Can you work these out from the drawing? Everything is in mm from the part's minimum corner. A direction names the side the tool comes from. Give positions to 0.01 mm unless a question says otherwise; leave off trailing zeros. Order: outer loops, then holes, each group sorted by start corner. A loop starts at its lowest first (then second) coordinate and runs counter-clockwise, first axis right, second up. Notation, with made-up numbers: (33.5, 45) - (62.5, 45) arc R20 ccw to (62.5, 76) - close; hole circle Ø4 at (17.25, 45). An arc over 180 degrees is marked (long way). One line per question, with ' | ' between items.
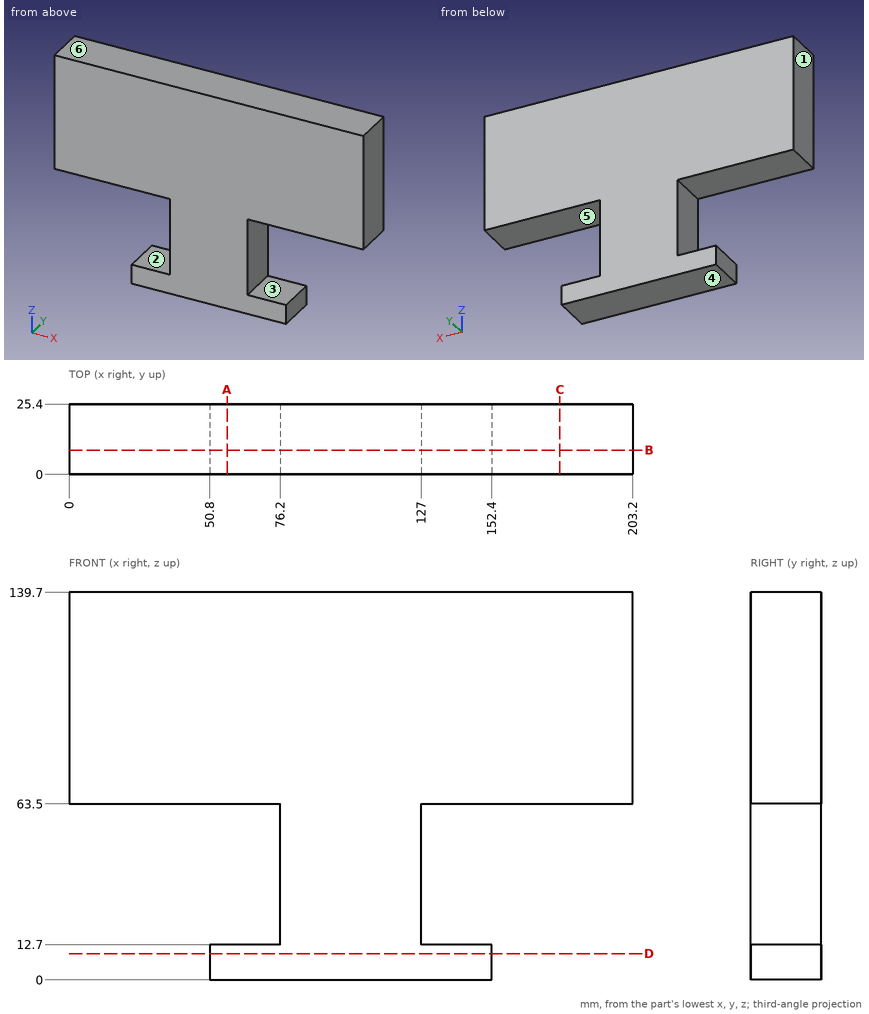
(1) Imagine slicing it at B-B (y = 8.75). List the corners of the cut face in (x, z) for me.
Answer below:
outline: (0, 63.5) - (76.2, 63.5) - (76.2, 12.7) - (50.8, 12.7) - (50.8, 0) - (152.4, 0) - (152.4, 12.7) - (127, 12.7) - (127, 63.5) - (203.2, 63.5) - (203.2, 139.7) - (0, 139.7) - close
(2) Imagine slicing it at A-A (x = 57). List the corners of the cut face in (y, z) for me.
Answer below:
outline: (0, 0) - (25.4, 0) - (25.4, 12.7) - (0, 12.7) - close; (0, 63.5) - (25.4, 63.5) - (25.4, 139.7) - (0, 139.7) - close
(3) If I drill on line 1 (Z direction, x = 141, y = 10.5); line 2 (Z direction, x = 169, y = 2.75); line 3 (X direction, y = 4.5, z = 30.5), over which ranges is the centre line in solid material (lowest first)?
Answer below:
line 1: 0 to 12.7, 63.5 to 139.7 | line 2: 63.5 to 139.7 | line 3: 76.2 to 127
(4) Imagine slicing it at D-D (z = 9.5). List the corners of the cut face in (x, y) for me.
Answer below:
outline: (50.8, 0) - (152.4, 0) - (152.4, 25.4) - (50.8, 25.4) - close
(5) On a 3-axis mill with a long thin cutter (end or side, diameter ignored), from which of +Z, -Z, +X, -X, +Y, -Y can I reach the whole of each face in a straight line? I mean the marked faces 1, 2 and 3. Say none if no direction works.
Answer below:
face 1: +Z, -Z, -X, +Y, -Y | face 2: -X, +Y, -Y | face 3: +X, +Y, -Y
(6) Will these pins go through, and if not, where does the flat tip stop? pin 1 (1 mm diameter, centred on y = 7, z = 45.5, fed in from -X); pin 2 (14 mm diameter, centred on y = 8, z = 4, fed in from -X); pin 3 (14 mm diameter, centred on y = 13, z = 9, fed in from +X).
Answer below:
pin 1: x = 76.2 | pin 2: x = 50.8 | pin 3: x = 152.4
(7) If we mould it in two halves opening along Z, with no side actions, what happens to the marked faces 4, 5 and 6? For each: released by +Z, released by -Z, zero draft, split by the parting line, or undercut.
Answer below:
face 4: released by -Z | face 5: undercut | face 6: released by +Z
(8) Imagine slicing it at C-C (x = 177). List the corners of the cut face in (y, z) for me.
Answer below:
outline: (0, 63.5) - (25.4, 63.5) - (25.4, 139.7) - (0, 139.7) - close
